```python
from build123d import *

# Parameters (mm, degrees)
SKETCH1_W            = 167.64
SKETCH1_H            = 109.22
PCB_DEPTH            = 1.5748
SKETCH2_R            = 1.75
MOUNT_HOLE_CUT_DEPTH = 1.5748
LPATTERN1_COUNT      = 2
LPATTERN1_PITCH      = 152.5
LPATTERN1_COUNT_DIR2 = 2
LPATTERN1_PITCH_DIR2 = 91.9
SKETCH3_W            = 7.463209877
SKETCH3_H            = 6.129068463
EXTRUDE1_DEPTH       = 3.75


with BuildPart() as part:
    # Sketch1 → PCB (new body)
    with BuildSketch(Plane.XY):
        with Locations((46.345343175, 16.988671329)):
            Rectangle(SKETCH1_W, SKETCH1_H)
    extrude(amount=PCB_DEPTH)

    # Sketch2 → mount hole cut (cut)
    with BuildSketch(Plane.XY.offset(1.5748)):
        with Locations((-29.854656825, 61.438671329)):
            Circle(SKETCH2_R)
    mount_hole_cut = extrude(amount=-MOUNT_HOLE_CUT_DEPTH, mode=Mode.SUBTRACT)

    # LPattern1: mount hole cut 2 × 2
    with Locations(*[(i * LPATTERN1_PITCH, -j * LPATTERN1_PITCH_DIR2, 0) for i in range(LPATTERN1_COUNT) for j in range(LPATTERN1_COUNT_DIR2) if (i, j) != (0, 0)]):
        add(mount_hole_cut, mode=Mode.SUBTRACT)

    # Sketch3 → Extrude1 (add)
    with BuildSketch(Plane(origin=(0, 0, 0), x_dir=(-1, 0, 0), z_dir=(0, 0, -1))):
        with Locations((7.354656825, -1.991328672)):
            Rectangle(SKETCH3_W, SKETCH3_H)
    extrude(amount=EXTRUDE1_DEPTH)


solid = part.part
```
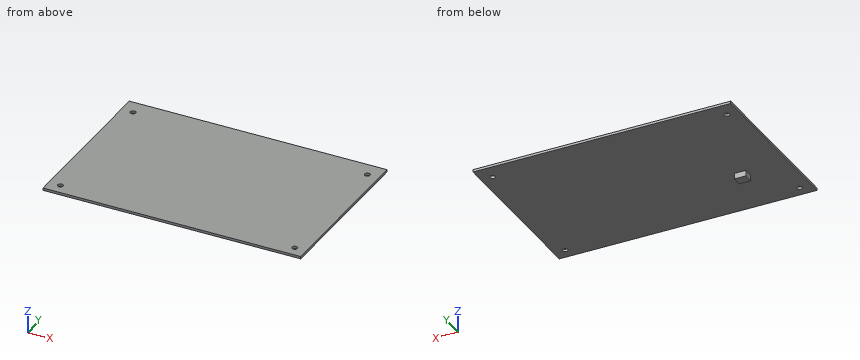
Build history of the part. All positions in model axes, mm. Give positions to 0.01 mm unless a question says otherwise; leave off trailing zeros. Loops run counter-clockwise (first coordinate to the right, second up) from the corner with the lowest first, then second, coordinate; pieces in that order, holes last.
Item 1: Slice it at B-B, the plane x = 79.5. List the corners of the cut face in (y, z).
Answers follow:
outline: (-37.62, 0) - (71.6, 0) - (71.6, 1.57) - (-37.62, 1.57) - close
Item 2: Drill centre lines: line 1 (X direction, y = 62.5, z = 0.35); line 2 (Z direction, x = 46, y = 42); line 3 (Y direction, x = -7.5, z = -1.8). Where is each one in solid material? Low to high.
Answers follow:
line 1: x = -37.47 to -31.25, -28.46 to 121.25, 124.04 to 130.17
line 2: z = 0 to 1.57
line 3: y = -5.06 to 1.07
Item 3: Flat gauge pins, fed straight in: pin 1 (5.5 mm diameter, centred on x = 122.65, y = 61.44, fed in from -Z); pin 2 (3 mm diameter, centred on y = -2.5, z = -2, fed in from +X); pin 3 (3 mm diameter, centred on y = -3.5, z = -2, fed in from -X). Where does each tip first touch, or does it go through?
Answers follow:
pin 1: stops at z = 0
pin 2: stops at x = -3.62
pin 3: stops at x = -11.09
Item 4: Slice it at A-A, the plane z = -2.9. List the corners of the cut face in (x, y).
Answers follow:
outline: (-11.09, -5.06) - (-3.62, -5.06) - (-3.62, 1.07) - (-11.09, 1.07) - close
